Design review of the part built by this model. Coordinates are the model's own, in mm. A direction names the side the tool comes from. Round coordinates to 2 decimals unless told otherwise and drop trailing zeros. Loops run counter-clockwise (first coordinate to the right, second up) from the corner with the lowest first, then second, coordinate; pieces in that order, holes last. Notation, with made-up numbers: (-3.75, 37) - (48.25, 37) arc R13 cw to (48.25, 42) - close; hole circle Ø5 at (64, 56). An arc over 180 degrees is marked (long way). Return JSON: item names as keys, results as strings. Group by question number.
from build123d import *

# Parameters (mm, degrees)
F1_DEPTH = 12
F2_R     = 1.75
F3_DEPTH = 7.001


with BuildPart() as f1:
    # F0 (on Front) → F1 (new body)
    with BuildSketch(Plane.XZ):
        with BuildLine():
            Line((-28.697127, 0), (-25.697127, 0))
            Line((-25.697127, 0), (-25.697127, 15))
            Line((-25.697127, 15), (-21.697127, 15))
            Line((-21.697127, 15), (-21.697127, 35))
            Line((-21.697127, 35), (-23.697127, 35))
            ThreePointArc((-23.697127, 35), (-24.404233, 34.707107), (-24.697127, 34))
            Line((-24.697127, 34), (-24.697127, 21))
            ThreePointArc((-24.697127, 21), (-24.99002, 20.292893), (-25.697127, 20))
            Line((-25.697127, 20), (-26.697127, 20))
            ThreePointArc((-26.697127, 20), (-28.11134, 19.414214), (-28.697127, 18))
            Line((-28.697127, 18), (-28.697127, 0))
        make_face()
    extrude(amount=F1_DEPTH)

    # F2 (on face) → F3 (cut, through all)
    with BuildSketch(Plane.YZ.offset(-21.697127)):
        with Locations((-6, 28)):
            Circle(F2_R)
    extrude(amount=-F3_DEPTH, mode=Mode.SUBTRACT)


solid = f1.part
Q1. Add section A-A, the plane y = -6. State the section outline as (x, z) points, plus the area to 3 significant figures.
Q2. Draft analysis for pull direction Y (two halves, no side actions). For faces 1 (the flat face through (-27, -6, 0)), 2 (the cylindrical face through (-23.18, -7.29, 29.18)), 3 (the flat face through (-25, -12, 18)), state which applies: pulls with the +Y half, pulls with the -Y half, needs draft (parallel to the pull), parting line crosses it, or undercut.
Q3. Insertion check: pin 1 Ø3.5 at (y, z) = (-6.5, 7) entering from +X; pin 2 Ø3 at (y, z) = (-10.5, 29.5) entering from -X; pin 3 Ø2 at (x, y) = (-23, -5) entering from -Z. Each pin has a flat end and moves straight along its axis. Give the tip position at first contact, or say it passes through.
Q4. For line 1 (Z direction, x = -23.15, y = -6); line 2 (X direction, y = -10.25, z = 28.5); line 3 (Z direction, x = -23.25, y = -9), list the stretches that pass through material, from the lowest coordinate up.
Q5. Tool access review of faces 4 (the flat face through (-24, -6, 15)), 5 (the flat face through (-26, -6, 20)), 6 (the flat face through (-25, 0, 18)): name each direction out of +Z, -Z, +X, -X, +Y, -Y from which nothing blocks a thin tool from reaching the whole face with its end or side.
Q6. Add section C-C, the plane x = -23. State the section outline as (y, z) points, plus the area to 3 significant figures.
Q7. Add section B-B, the plane z = 28. State the section outline as (x, y) points.
Q8. Add section D-D, the plane y = -1.75. State the section outline as (x, z) points.
Evaluation:
{
 "1": {"outline": "(-28.7, 0) - (-25.7, 0) - (-25.7, 15) - (-21.7, 15) - (-21.7, 26.25) - (-24.7, 26.25) - (-24.7, 21) arc R1 cw to (-25.7, 20) - (-26.7, 20) arc R2 ccw to (-28.7, 18) - close; (-24.7, 29.75) - (-21.7, 29.75) - (-21.7, 35) - (-23.7, 35) arc R1 ccw to (-24.7, 34) - close", "area": "114 mm²"},
 "2": {"face 1": "needs draft", "face 2": "undercut", "face 3": "pulls with the -Y half"},
 "3": {"pin 1": "x = -25.7", "pin 2": "x = -24.7", "pin 3": "z = 15"},
 "4": {"line 1": "15 to 26.25, 29.75 to 35", "line 2": "-24.7 to -21.7", "line 3": "15 to 35"},
 "5": {"face 4": "-Z, +X, +Y, -Y", "face 5": "+Z, -X, +Y, -Y", "face 6": "+Z, -Z, +X, -X, +Y"},
 "6": {"outline": "(-12, 15) - (0, 15) - (0, 35) - (-12, 35) - close; hole circle Ø3.5 at (-6, 28)", "area": "230 mm²"},
 "7": {"outline": "(-24.7, -12) - (-21.7, -12) - (-21.7, -7.75) - (-24.7, -7.75) - close; (-24.7, -4.25) - (-21.7, -4.25) - (-21.7, 0) - (-24.7, 0) - close"},
 "8": {"outline": "(-28.7, 0) - (-25.7, 0) - (-25.7, 15) - (-21.7, 15) - (-21.7, 35) - (-23.7, 35) arc R1 ccw to (-24.7, 34) - (-24.7, 21) arc R1 cw to (-25.7, 20) - (-26.7, 20) arc R2 ccw to (-28.7, 18) - close"}
}
